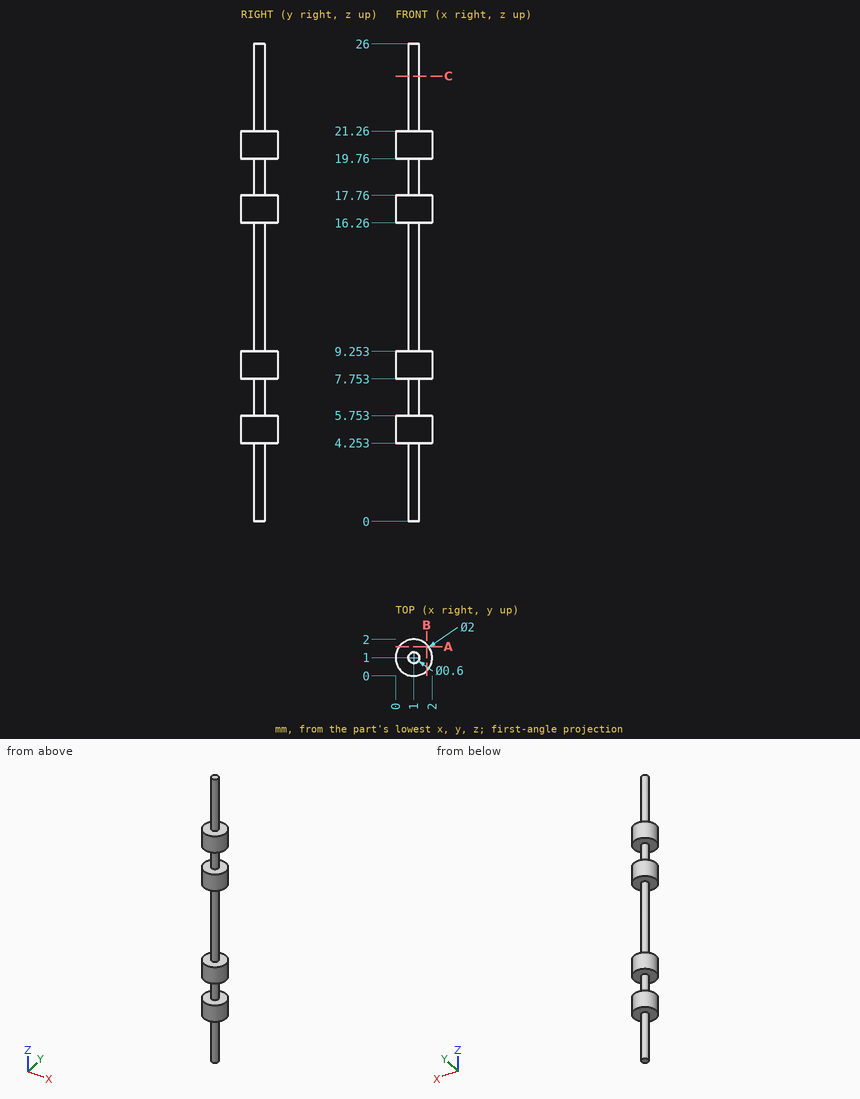
Geometry: see drawing. Coordinates: mm, zero at the bounding-box minimum. Give positions to 0.01 mm unless a question says otherwise; leave off trailing zeros. Write each loop counter-clockwise with the first axis right and the second up, starting at its lowest first coordinate (ties: lowest second). Pieces come first, ordered by that corner, then holes. Notation, with made-up numbers: (-33.75, 17) - (-8.75, 17) arc R9 ccw to (-8.75, 29) - close; hole circle Ø11 at (38.5, 48.5). An arc over 180 degrees is marked (long way). Return JSON: item names as keys, results as strings. Group by question number.
1) First-contact query: P1, Ø1, axis at x = 1, y = 1.5, coming from the -Z side; P2, Ø1, axis at x = 0, z = 13, coming from the +Y side; P3, Ø1, axis at y = 1.5, z = 4, coming from the -X side. Flat tips, straight axial feed; report the tip coordinate or a pass-through.
2) Section C-C on z = 24.25. Return the cut outline in (x, y).
3) Section B-B on x = 1.7. Return the cut outline in (y, z).
4) Section A-A on y = 1.6. Return the cut outline in (x, z).
5) Line query: line 1 (Z direction, x = 0.8, y = 1.65); line 2 (X direction, y = 0.95, z = 11); line 3 (X direction, y = 0.75, z = 14). Output: solid intervals per line, ascending.
Filled in:
{
 "1": {"P1": "stops at z = 0", "P2": "passes through", "P3": "stops at x = 0"},
 "2": {"outline": "circle Ø0.6 at (1, 1)"},
 "3": {"outline": "(0.29, 4.25) - (1.71, 4.25) - (1.71, 5.75) - (0.29, 5.75) - close; (0.29, 7.75) - (1.71, 7.75) - (1.71, 9.25) - (0.29, 9.25) - close; (0.29, 16.26) - (1.71, 16.26) - (1.71, 17.76) - (0.29, 17.76) - close; (0.29, 19.76) - (1.71, 19.76) - (1.71, 21.26) - (0.29, 21.26) - close"},
 "4": {"outline": "(0.2, 4.25) - (1.8, 4.25) - (1.8, 5.75) - (0.2, 5.75) - close; (0.2, 7.75) - (1.8, 7.75) - (1.8, 9.25) - (0.2, 9.25) - close; (0.2, 16.26) - (1.8, 16.26) - (1.8, 17.76) - (0.2, 17.76) - close; (0.2, 19.76) - (1.8, 19.76) - (1.8, 21.26) - (0.2, 21.26) - close"},
 "5": {"line 1": "z = 4.25 to 5.75, 7.75 to 9.25, 16.26 to 17.76, 19.76 to 21.26", "line 2": "x = 0.7 to 1.3", "line 3": "x = 0.83 to 1.17"}
}
